```python
from build123d import *

# Parameters (mm, degrees)
SKETCH1_R           = 4
SKETCH1_W           = 10
SKETCH1_H           = 50
BOSS_EXTRUDE1_DEPTH = 7.5
SKETCH3_W           = 10
SKETCH3_H           = 25
SKETCH3_W_2         = 20
SKETCH3_H_2         = 80
SKETCH3_H_3         = 50
BOSS_EXTRUDE2_DEPTH = 25
LPATTERN1_COUNT     = 2
LPATTERN1_PITCH     = 32.5
SKETCH4_R           = 12.5
CUT_EXTRUDE1_DEPTH  = 3
SKETCH4_3_R         = 5
CUT_EXTRUDE2_DEPTH  = 40
SKETCH4_4_R         = 2.5
CUT_EXTRUDE3_DEPTH  = 4
SKETCH5_R           = 5
CUT_EXTRUDE4_DEPTH  = 5


with BuildPart() as part:
    # Sketch1 → Boss-Extrude1 (new body)
    with BuildSketch(Plane(origin=(0, -20, 0), x_dir=(1, 0, 0), z_dir=(0, 1, 0))):
        with BuildLine():
            Line((0, 40), (0, -40))
            Line((0, -40), (25, -40))
            Line((25, -40), (70.319765879, -69.141388534))
            ThreePointArc((70.319765879, -69.141388534), (78.074234717, -70.981200492), (85.271064581, -67.557410938))
            Line((85.271064581, -67.557410938), (101.461064602, -51.459429229))
            ThreePointArc((101.461064602, -51.459429229), (104.079999441, -47.5579944), (105, -42.95))
            Line((105, -42.95), (105, 42.95))
            ThreePointArc((105, 42.95), (104.079999441, 47.5579944), (101.461064602, 51.459429229))
            Line((101.461064602, 51.459429229), (85.271064581, 67.557410938))
            ThreePointArc((85.271064581, 67.557410938), (78.074234717, 70.981200492), (70.319765879, 69.141388534))
            Line((70.319765879, 69.141388534), (25, 40))
            Line((25, 40), (0, 40))
        make_face()
        with Locations(Location((78.7, -62.5, 0), (0, 0, 270))):
            Circle(SKETCH1_R, mode=Mode.SUBTRACT)
        with Locations(Location((95.05, -42.95, 0), (0, 0, 270))):
            Circle(SKETCH1_R, mode=Mode.SUBTRACT)
        with Locations(Location((95.05, 42.95, 0), (0, 0, 90))):
            Circle(SKETCH1_R, mode=Mode.SUBTRACT)
        with Locations(Location((78.7, 62.5, 0), (0, 0, 90))):
            Circle(SKETCH1_R, mode=Mode.SUBTRACT)
        with Locations((9, 0)):
            Rectangle(SKETCH1_W, SKETCH1_H, mode=Mode.SUBTRACT)
        Polygon((30.85, -31.872701463), (30.85, 31.872701463), (69.747715914, 56.88460147), (85, 41.719006045), (85, -41.719006045), (69.747715914, -56.88460147), align=None, mode=Mode.SUBTRACT)
    boss_extrude1 = extrude(amount=BOSS_EXTRUDE1_DEPTH)

    # Sketch3 → Boss-Extrude2 (add)
    # profile 1 of 2: a face of its own
    with BuildSketch(Plane(origin=(0, -12.5, 0), x_dir=(1, 0, 0), z_dir=(0, 1, 0))):
        with Locations((100, 0)):
            Rectangle(SKETCH3_W, SKETCH3_H)
    # profile 2 of 2: a face of its own
    with BuildSketch(Plane(origin=(0, -12.5, 0), x_dir=(1, 0, 0), z_dir=(0, 1, 0))):
        with Locations((10, 0)):
            Rectangle(SKETCH3_W_2, SKETCH3_H_2)
        with Locations((9, 0)):
            Rectangle(SKETCH3_W, SKETCH3_H_3, mode=Mode.SUBTRACT)
    extrude(amount=BOSS_EXTRUDE2_DEPTH)

    # LPattern1: Boss-Extrude1 ×2
    with Locations(*[(0, i * LPATTERN1_PITCH, 0) for i in range(1, LPATTERN1_COUNT)]):
        add(boss_extrude1)

    # Sketch4 → Cut-Extrude1 (cut)
    with BuildSketch(Plane.ZY):
        Circle(SKETCH4_R)
    extrude(amount=-CUT_EXTRUDE1_DEPTH, mode=Mode.SUBTRACT)

    # Sketch4_3 → Cut-Extrude2 (cut)
    with BuildSketch(Plane.ZY):
        Circle(SKETCH4_3_R)
    extrude(amount=-CUT_EXTRUDE2_DEPTH, mode=Mode.SUBTRACT)

    # Sketch4_4 → Cut-Extrude3 (cut)
    with BuildSketch(Plane.ZY):
        with Locations((15.5, 15.5)):
            Circle(SKETCH4_4_R)
        with Locations((-15.5, 15.5)):
            Circle(SKETCH4_4_R)
        with Locations((-15.5, -15.5)):
            Circle(SKETCH4_4_R)
        with Locations((15.5, -15.5)):
            Circle(SKETCH4_4_R)
    extrude(amount=-CUT_EXTRUDE3_DEPTH, mode=Mode.SUBTRACT)

    # Sketch5 → Cut-Extrude4 (cut)
    with BuildSketch(Plane.ZY.offset(-95)):
        Circle(SKETCH5_R)
    extrude(amount=-CUT_EXTRUDE4_DEPTH, mode=Mode.SUBTRACT)


solid = part.part
```
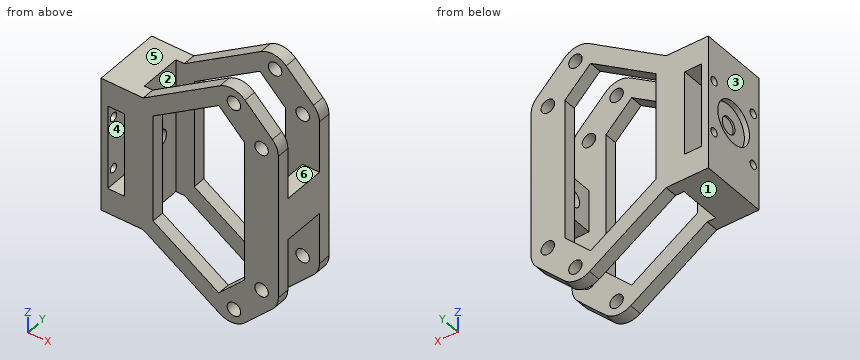
Design review of the part built by this model. Coordinates are the model's own, in mm. Face numbers are marked on the shaded views. A direction names the side the tool comes from. Round coordinates to 2 decimals unless told otherwise and drop trailing zeros. Order: outer loops, then holes, each group sorted by start corner. A loop starts at its lowest first (then second) coordinate and runs counter-clockwise, first axis right, second up. Notation, with made-up numbers: M 5.5,65 L 43.5,65 A18 cw 43.5,84 Z; hole C 33.25,12.5 d1. An arc over 180 degrees is marked long. Put each result on its own line as item: value.
Q1. To check wall thickness, follow line 1 (Y direction, x = 3.05, z = -15.5); line 2 (X direction, y = -17.5, z = 9.5); line 3 (Y direction, x = 75, z = -65). State the ranges of each line that lie inside material, in increasing order.
Reported:
line 1: -20 to -18, -13 to 13, 18 to 20
line 2: 0 to 4, 14 to 30.85, 85 to 105
line 3: -20 to -12.5, 12.5 to 20
Q2. Consider section D-D (y = -7.5). State the section outline as (x, z) points, and give its area (3 significant figures).
Reported:
outline: M 0,-40 L 20,-40 L 20,40 L 0,40 L 0,10 L 3,10 L 3,-10 L 0,-10 Z; M 95,-12.5 L 105,-12.5 L 105,12.5 L 95,12.5 Z; hole M 4,-25 L 14,-25 L 14,25 L 4,25 Z
area: 1,290 mm²
Q3. Consider section A-A (y = 15.5). State how many separate pieces and enclosed holes the cut face has, and give its area (3 significant figures).
Reported:
separate pieces: 2
enclosed holes: 5
area: 5,620 mm²
Q4. Draft analysis for pull direction X (two halves, no side actions). For the marked faces 1, 2 and 3, state which applies: released by +X, released by -X, zero draft, split by the parting line, or undercut.
Reported:
face 1: zero draft
face 2: undercut
face 3: released by -X
Q5. Consider section C-C (y = 0). State the section outline as (x, z) points, and give its area (4 significant figures).
Reported:
outline: M 0,-40 L 20,-40 L 20,-5 L 14,-5 L 14,-25 L 4,-25 L 4,-5 L 3,-5 L 3,-12.5 L 0,-12.5 Z; M 0,12.5 L 3,12.5 L 3,5 L 4,5 L 4,25 L 14,25 L 14,5 L 20,5 L 20,40 L 0,40 Z; M 95,-12.5 L 105,-12.5 L 105,12.5 L 95,12.5 L 95,5 L 100,5 L 100,-5 L 95,-5 Z
area: 1,155 mm²
Q6. Consider section B-B (x = 10.5). State the section outline as (y, z) points, and give its area (3 significant figures).
Reported:
outline: M -20,-40 L 20,-40 L 20,-25 L -20,-25 Z; M -20,25 L 20,25 L 20,40 L -20,40 Z
area: 1,200 mm²
Q7. Insertion check: pin 1 Ø5 at (x, y) = (15.5, 12) entering from +Z; pin 2 Ø4 at (y, z) = (-15.5, -15.5) entering from -X; pin 3 Ø20 at (y, z) = (-0.5, 1.5) entering from -X. Each pin has a flat end and moves straight along its axis. Give the tip position at first contact, or say it passes through.
Reported:
pin 1: z = 40
pin 2: x = 14
pin 3: x = 3
Q8. Machinability: for the marked faces 4, 5 and 6, which of the approach directions +Z, -Z, +X, -X, +Y, -Y give a long, thin tool a straight path to every point of the face, cutting with its end or side? Answer none if there is none.
Reported:
face 4: +Y, -Y
face 5: +Z, -X, +Y, -Y
face 6: +Z, +X
